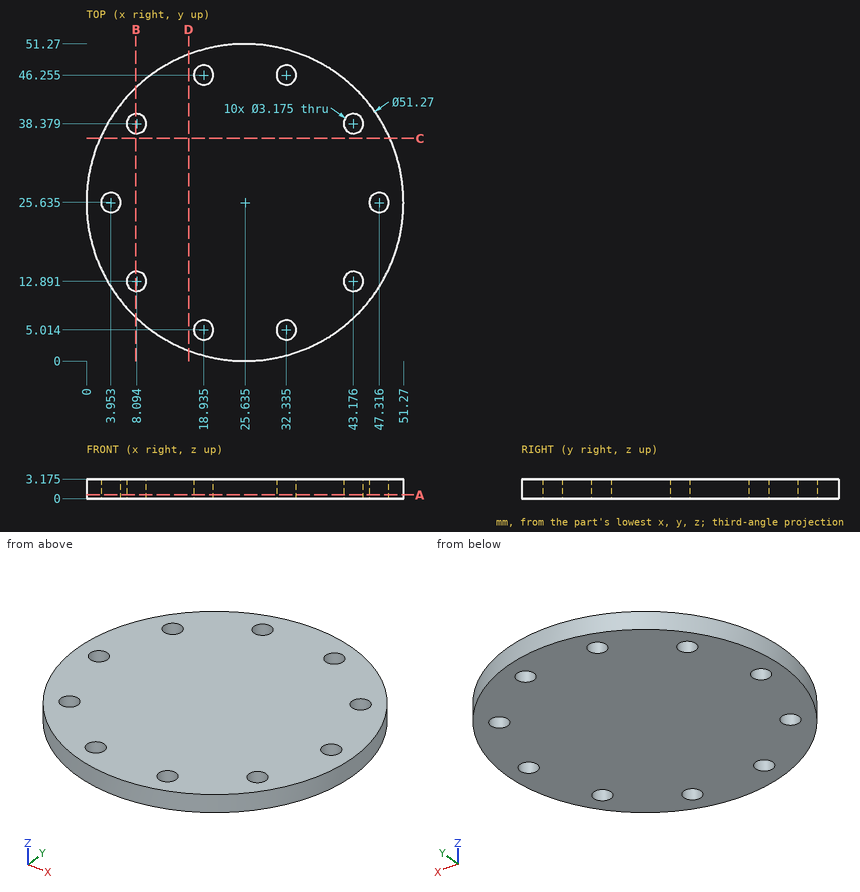
Study the drawing (mm; zero at the part's minimum x, y, z) and answer. Give positions to 0.01 mm unless a question says otherwise; leave off trailing zeros. Loops run counter-clockwise (first coordinate to the right, second up) from the corner with the lowest first, then second, coordinate; pieces in that order, holes last. Notation, with made-up numbers: M 66,64.25 L 88,64.25 A32 cw 88,91.25 Z; hole C -16,36.25 d5. An arc over 180 degrees is marked long. One line per item, written item: value. Start each with the question number.
1. Find section C-C (y = 36). Give the vertices of the cut face in (x, z) (1 decimal), and give its area (3 significant figures).
2. Find the intervals of material crossed by probe 1 along Y at (x, z) = (18.5, 1.6); probe 2 along X at (y, z) = (13, 1.8); probe 3 along Y at (x, z) = (31, 3) (1 decimal), in increasing order.
3. Find section B-B (x = 8). Give the vertices of the cut face in (y, z) (1 decimal).
4. Find section D-D (x = 16.5). Give the vertices of the cut face in (y, z) (1 decimal).
5. Find section A-A (z = 0.6). State how many separate pieces and enclosed holes the cut face has, and give its area (3 significant figures).
6. This flat-tipped pin is pushed along its axis until it touches: P1, Ø1.5, axis at x = 42.5, z = 2.5, coming from the +Y side. Where does it stop, or does it pass through?
Reported:
1. outline: M 2.2,0 L 49.1,0 L 49.1,3.2 L 2.2,3.2 Z
1. area: 149 mm²
2. probe 1: y = 1.01 to 3.49, 6.54 to 44.73, 47.78 to 50.26
2. probe 2: x = 3.33 to 6.51, 9.68 to 41.59, 44.76 to 47.94
2. probe 3: y = 0.6 to 4.2, 5.9 to 45.4, 47.1 to 50.7
3. outline: M 7,0 L 11.3,0 L 11.3,3.2 L 7,3.2 Z; M 14.5,0 L 36.8,0 L 36.8,3.2 L 14.5,3.2 Z; M 40,0 L 44.2,0 L 44.2,3.2 L 40,3.2 Z
4. outline: M 1.7,0 L 49.6,0 L 49.6,3.2 L 1.7,3.2 Z
5. separate pieces: 1
5. enclosed holes: 10
5. area: 1,990 mm²
6. P1: stops at y = 45.57
